```python
from build123d import *
from OCP.BRepFilletAPI import BRepFilletAPI_MakeFillet

# Parameters (mm, degrees)
SKETCH1_R           = 2.6
BOSS_EXTRUDE1_DEPTH = 26
SKETCH2_W           = 18
SKETCH2_H           = 20
CUT_EXTRUDE1_DEPTH  = 5
CUT_EXTRUDE2_START  = 26
SKETCH3_W           = 18
SKETCH3_H           = 38
CUT_EXTRUDE2_DEPTH  = 18
CUT_EXTRUDE3_START  = 18.5
SKETCH4_R           = 1.4
CUT_EXTRUDE3_DEPTH  = 10
FILLET1_R           = 4
FILLET1_R_2         = 2
CUT_EXTRUDE4_DEPTH  = 2
SKETCH6_W           = 37
SKETCH6_H           = 16
BOSS_EXTRUDE2_DEPTH = 8
FILLET2_R           = 15
SKETCH7_R           = 1.5
CUT_EXTRUDE5_DEPTH  = 22


with BuildPart() as part:
    # Sketch1 → Boss-Extrude1 (new body)
    with BuildSketch(Plane.XY):
        Polygon((-13, -13.5), (13, -13.5), (13, 18.5), (-3, 18.5), (-3, 24.5), (-13, 24.5), (-13, 13.5), align=None)
        with Locations(Location((-8, 19.25, 0), (0, 0, 180))):
            Circle(SKETCH1_R, mode=Mode.SUBTRACT)
        with Locations(Location((-8, 9.25, 0), (0, 0, 180))):
            Circle(SKETCH1_R, mode=Mode.SUBTRACT)
    extrude(amount=BOSS_EXTRUDE1_DEPTH)

    # Sketch2 → Cut-Extrude1 (cut)
    with BuildSketch(Plane.XY):
        with Locations((-4, 14.5)):
            Rectangle(SKETCH2_W, SKETCH2_H)
    extrude(amount=CUT_EXTRUDE1_DEPTH, mode=Mode.SUBTRACT)

    # Sketch3 → Cut-Extrude2 (cut)
    with BuildSketch(Plane.XY.offset(CUT_EXTRUDE2_START)):
        with Locations((-4, 5.5)):
            Rectangle(SKETCH3_W, SKETCH3_H)
    extrude(amount=-CUT_EXTRUDE2_DEPTH, mode=Mode.SUBTRACT)

    # Sketch4 → Cut-Extrude3 (cut)
    with BuildSketch(Plane(origin=(0, 0, 0), x_dir=(1, 0, 0), z_dir=(0, 1, 0)).offset(CUT_EXTRUDE3_START)):
        with Locations(Location((9, -11, 0), (0, 0, 270))):
            Circle(SKETCH4_R)
        with Locations(Location((9, -21, 0), (0, 0, 270))):
            Circle(SKETCH4_R)
    extrude(amount=-CUT_EXTRUDE3_DEPTH, mode=Mode.SUBTRACT)

    # Fillet1
    fillet1_edges_1 = [part.edges().sort_by_distance(p)[0] for p in [
        (-3, 24.5, 6.5),
        (-13, 24.5, 6.5),
        (5, 11.5, 5),
        (5, 2.5, 8),
        (5, 2.5, 26),
    ]]
    fillet1_edges_2 = [part.edges().sort_by_distance(p)[0] for p in [
        (-3, 18.5, 6.5),
    ]]
    fillet1 = BRepFilletAPI_MakeFillet(part.part.solid().wrapped)
    for e in fillet1_edges_1:
        fillet1.Add(FILLET1_R - 0.0001, e.wrapped)
    for e in fillet1_edges_2:
        fillet1.Add(FILLET1_R_2 - 0.0001, e.wrapped)
    add(Compound.cast(fillet1.Shape()), mode=Mode.REPLACE)  # a hair under: the kernel refuses the full size

    # Sketch5 → Cut-Extrude4 (cut)
    with BuildSketch(Plane.XY):
        with BuildLine():
            Line((-8, -5.85), (-13, -5.85))
            Line((-13, -5.85), (-13, 4.5))
            Line((-13, 4.5), (-8, 4.5))
            Line((-8, 4.5), (-2.9, 4.5))
            Line((-2.9, 4.5), (-2.9, -0.75))
            ThreePointArc((-2.9, -0.75), (-4.393755416, -4.356244584), (-8, -5.85))
        make_face()
    extrude(amount=CUT_EXTRUDE4_DEPTH, mode=Mode.SUBTRACT)

    # Sketch6 → Boss-Extrude2 (add)
    with BuildSketch(Plane.XY):
        with Locations((-17.5, -21.5)):
            Rectangle(SKETCH6_W, SKETCH6_H)
    extrude(amount=BOSS_EXTRUDE2_DEPTH)

    # Fillet2
    fillet2_edges = [part.edges().sort_by_distance(p)[0] for p in [
        (-13, -13.5, 4),
        (1, -29.5, 4),
    ]]
    fillet(fillet2_edges, radius=FILLET2_R)

    # Sketch7 → Cut-Extrude5 (cut)
    with BuildSketch(Plane.XY):
        with Locations(Location((-20.052596491, -17.5, 0), (0, 0, 180))):
            Circle(SKETCH7_R)
        with Locations(Location((-27.052596491, -23, 0), (0, 0, 180))):
            Circle(SKETCH7_R)
    extrude(amount=CUT_EXTRUDE5_DEPTH, mode=Mode.SUBTRACT)


solid = part.part
```
Geometry check sheet. Reference: the model listing, model coordinates, mm. A direction names the side the tool comes from. Give positions to 0.01 mm unless a question says otherwise; leave off trailing zeros. Order: outer loops, then holes, each group sorted by start corner. A loop starts at its lowest first (then second) coordinate and runs counter-clockwise, first axis right, second up. Notation, with made-up numbers: (45, 29.5) - (57, 29.5) arc R24 ccw to (57, 48.5) - close; hole circle Ø4 at (70.5, 35.25). An arc over 180 degrees is marked (long way). Answer in a Markdown table with one row per item. Add a question column.
Q1. Cross-section at A-A, the plane y = 9.25. Enter the section's corners in (x, z).
Q2. Gauge pin test, flat ends, axial feed: pin 1 (11 mm diameter, centred on y = -1.5, z = 19, fed in from -X); pin 2 (5 mm diameter, centred on y = 7, z = 4.5, fed in from -X); pin 3 (5 mm diameter, centred on x = -20.05, y = -17.5, fed in from +Z); pin 4 (1.8 mm diameter, centred on x = -27.05, y = -23, fed in from -Z). Record the tip position at first contact, or that the pin passes through.
Q3. Cross-section at B-B, the plane z = 21. Enter the section's corners in (x, y).
Q4. Tool access check on faces 1 (the flat face through (-32, -13.5, 4)), 2 (the flat face through (9, 8.5, 11)), 3 (the cylindrical face through (-4.354, -4.316, 0.986)), 4 (the flat face through (9, 18.5, 13)). Record the directions out of +Z, -Z, +X, -X, +Y, -Y that give a thin tool (end or side, any length) a straight path to the whole face; none if there is none.
Q5. Cross-section at C-C, the plane x = 2. Enter the section's corners in (y, z), then the cut area to 3 significant figures.
Q6. Mould release check, pull along X, two halves, no side actions. Record for faces 5 (the flat face through (-12, -16, 0)), 6 (the cylindrical face through (-26.857, -24.487, 3.944)), 7 (the flat face through (-13, 11, 6)), 8 (the cylindrical face through (-3.51, -25.22, 4.06)): pulls with the +X half, pulls with the -X half, needs draft (parallel to the pull), parting line crosses it, or undercut.
Q7. Cross-section at D-D, the plane z = 11. Enter the section's corners in (x, y), then the cut area to 3 significant figures.
Q8. Material ranges on probe 1 along Z at (x, y) = (-21.5, -19); probe 2 along Y at (x, z) = (10.5, 21.5); probe 3 along X at (y, z) = (16.5, 21), recorded low to high. Write a range as from..to.
Check values:
| question | item | result |
|---|---|---|
| 1 | outline | (-13, 5) - (-10.6, 5) - (-10.6, 8) - (-13, 8) - close; (-5.4, 5) - (1, 5) arc R4 cw to (5, 1) - (5, 0) - (13, 0) - (13, 26) - (9, 26) arc R4 ccw to (5, 22) - (5, 12) arc R4 cw to (1, 8) - (-5.4, 8) - close; hole circle Ø2.8 at (9, 11); hole circle Ø2.8 at (9, 21) |
| 2 | pin 1 | stops at x = 5 |
| 2 | pin 2 | stops at x = -13 |
| 2 | pin 3 | stops at z = 8 |
| 2 | pin 4 | passes through |
| 3 | outline | (5, -13.5) - (13, -13.5) - (13, 18.5) - (10.4, 18.5) - (10.4, 8.5) - (7.6, 8.5) - (7.6, 18.5) - (5, 18.5) - close |
| 4 | face 1 | +Z, -Z, -X, +Y |
| 4 | face 2 | +Y |
| 4 | face 3 | -Z, -X, +Y |
| 4 | face 4 | +Z, -Z, +X, +Y |
| 5 | outline | (-13.5, 0) - (4.5, 0) - (4.5, 4.87) - (18.5, 4.87) - (18.5, 8.13) - (-13.5, 8.13) - close |
| 5 | area | 192 mm^2 |
| 6 | face 5 | needs draft |
| 6 | face 6 | undercut |
| 6 | face 7 | pulls with the -X half |
| 6 | face 8 | pulls with the +X half |
| 7 | outline | (4.87, -13.5) - (13, -13.5) - (13, 18.5) - (10.4, 18.5) - (10.4, 8.5) - (7.6, 8.5) - (7.6, 18.5) - (4.87, 18.5) - close |
| 7 | area | 232 mm^2 |
| 8 | probe 1 | z = 0..8 |
| 8 | probe 2 | y = -13.5..18.5 |
| 8 | probe 3 | x = 5..7.6, 10.4..13 |
